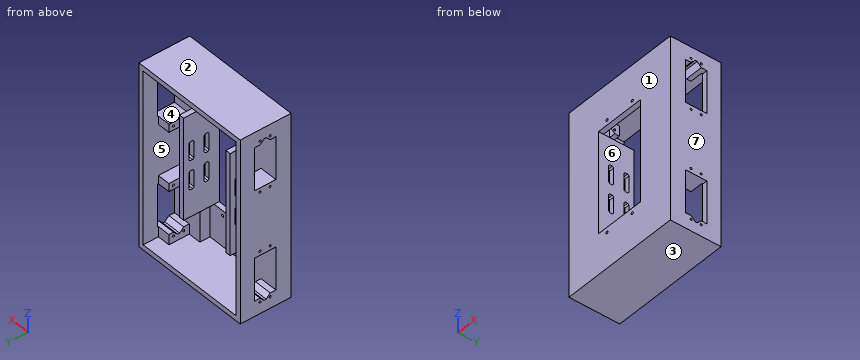
```python
from build123d import *

# Parameters (mm, degrees)
SKETCH1_W               = 120
SKETCH1_H               = 180
BOSS_EXTRUDE1_DEPTH     = 50
SHELL1_T                = -5
SKETCH2_W               = 5
SKETCH2_H               = 100
BOSS_EXTRUDE2_DEPTH     = 30
SKETCH3_W               = 25
SKETCH3_H               = 60
BOSS_EXTRUDE3_DEPTH     = 30
CUT_EXTRUDE1_REACH      = 224.036
SKETCH4_R               = 1
SKETCH5_W               = 12.5
SKETCH5_H               = 60
CUT_EXTRUDE2_DEPTH      = 20
CUT_EXTRUDE4_DEPTH      = 10
SKETCH6_R               = 1.25
SKETCH6_W               = 50
SKETCH6_H               = 100
CUT_EXTRUDE3_DEPTH      = 10
MIRROR2_COPY_1_SKETCH_W = 25
MIRROR2_COPY_1_SKETCH_H = 60
MIRROR2_COPY_1_DEPTH    = 30
MIRROR2_COPY_2_REACH    = 224.036
MIRROR2_COPY_2_SKETCH_R = 1
MIRROR2_COPY_3_SKETCH_W = 12.5
MIRROR2_COPY_3_SKETCH_H = 60
MIRROR2_COPY_3_DEPTH    = 20
MIRROR2_COPY_4_DEPTH    = 10


with BuildPart() as part:
    # Sketch1 → Boss-Extrude1 (new body)
    with BuildSketch(Plane(origin=(0, 0, 0), x_dir=(1, 0, 0), z_dir=(0, 1, 0))):
        with Locations((0, 90)):
            Rectangle(SKETCH1_W, SKETCH1_H)
    extrude(amount=BOSS_EXTRUDE1_DEPTH)

    # Shell1
    shell1_openings = [part.faces().sort_by_distance(p)[0] for p in [
        (0, 50, -90),
    ]]
    offset(amount=SHELL1_T, openings=shell1_openings, kind=Kind.INTERSECTION)

    # Sketch2 → Boss-Extrude2 (add)
    with BuildSketch(Plane(origin=(0, 5, 0), x_dir=(1, 0, 0), z_dir=(0, 1, 0))):
        with Locations((-27.5, 90)):
            Rectangle(SKETCH2_W, SKETCH2_H)
        with Locations((27.5, 90)):
            Rectangle(SKETCH2_W, SKETCH2_H)
    extrude(amount=BOSS_EXTRUDE2_DEPTH)

    # Sketch3 → Boss-Extrude3 (add)
    with BuildSketch(Plane(origin=(0, 5, 0), x_dir=(1, 0, 0), z_dir=(0, 1, 0))):
        with Locations((-42.5, 35)):
            Rectangle(SKETCH3_W, SKETCH3_H)
    boss_extrude3 = extrude(amount=BOSS_EXTRUDE3_DEPTH)

    # Cut-Extrude1: up to this face of the body (flat: up to its plane)
    cut_extrude1_end = Plane(part.part.faces().sort_by_distance((-30, 20, -102.5))[0])
    # Sketch4 → Cut-Extrude1 (cut, up to the picked face)
    with BuildSketch(Plane.ZY.offset(60), mode=Mode.PRIVATE) as cut_extrude1_sk1:
        with Locations((-61, 30.5)):
            Circle(SKETCH4_R)
    cut_extrude1_tool1 = split(extrude(cut_extrude1_sk1.sketch, amount=-CUT_EXTRUDE1_REACH, mode=Mode.PRIVATE), bisect_by=cut_extrude1_end, keep=Keep.BOTH, mode=Mode.PRIVATE)
    # Sketch4 → Cut-Extrude1 (cut, up to the picked face)
    with BuildSketch(Plane.ZY.offset(60), mode=Mode.PRIVATE) as cut_extrude1_sk2:
        with Locations((-61, 20.5)):
            Circle(SKETCH4_R)
    cut_extrude1_tool2 = split(extrude(cut_extrude1_sk2.sketch, amount=-CUT_EXTRUDE1_REACH, mode=Mode.PRIVATE), bisect_by=cut_extrude1_end, keep=Keep.BOTH, mode=Mode.PRIVATE)
    # Sketch4 → Cut-Extrude1 (cut, up to the picked face)
    with BuildSketch(Plane.ZY.offset(60), mode=Mode.PRIVATE) as cut_extrude1_sk3:
        with Locations((-11.220773398, 30.5)):
            Circle(SKETCH4_R)
    cut_extrude1_tool3 = split(extrude(cut_extrude1_sk3.sketch, amount=-CUT_EXTRUDE1_REACH, mode=Mode.PRIVATE), bisect_by=cut_extrude1_end, keep=Keep.BOTH, mode=Mode.PRIVATE)
    # Sketch4 → Cut-Extrude1 (cut, up to the picked face)
    with BuildSketch(Plane.ZY.offset(60), mode=Mode.PRIVATE) as cut_extrude1_sk4:
        with Locations((-11.220773398, 20.5)):
            Circle(SKETCH4_R)
    cut_extrude1_tool4 = split(extrude(cut_extrude1_sk4.sketch, amount=-CUT_EXTRUDE1_REACH, mode=Mode.PRIVATE), bisect_by=cut_extrude1_end, keep=Keep.BOTH, mode=Mode.PRIVATE)
    # Sketch4 → Cut-Extrude1 (cut, up to the picked face)
    with BuildSketch(Plane.ZY.offset(60), mode=Mode.PRIVATE) as cut_extrude1_sk5:
        Polygon((-57, 15), (-15, 15), (-15, 20.5), (-11, 24.5), (-11, 26.5), (-15, 30.5), (-15, 36), (-57, 36), align=None)
    cut_extrude1_tool5 = split(extrude(cut_extrude1_sk5.sketch, amount=-CUT_EXTRUDE1_REACH, mode=Mode.PRIVATE), bisect_by=cut_extrude1_end, keep=Keep.BOTH, mode=Mode.PRIVATE)
    cut_extrude1_1 = cut_extrude1_tool1.solids().sort_by(Axis((-60, 30.5, -61), (1, 0, 0)))[0]
    add(cut_extrude1_1, mode=Mode.SUBTRACT)
    cut_extrude1_2 = cut_extrude1_tool2.solids().sort_by(Axis((-60, 20.5, -61), (1, 0, 0)))[0]
    add(cut_extrude1_2, mode=Mode.SUBTRACT)
    cut_extrude1_3 = cut_extrude1_tool3.solids().sort_by(Axis((-60, 30.5, -11.220773), (1, 0, 0)))[0]
    add(cut_extrude1_3, mode=Mode.SUBTRACT)
    cut_extrude1_4 = cut_extrude1_tool4.solids().sort_by(Axis((-60, 20.5, -11.220773), (1, 0, 0)))[0]
    add(cut_extrude1_4, mode=Mode.SUBTRACT)
    cut_extrude1_5 = cut_extrude1_tool5.solids().sort_by(Axis((-60, 25.5, -35.402502), (1, 0, 0)))[0]
    add(cut_extrude1_5, mode=Mode.SUBTRACT)
    cut_extrude1 = cut_extrude1_1 + cut_extrude1_2 + cut_extrude1_3 + cut_extrude1_4 + cut_extrude1_5  # Cut-Extrude1 as one shape, for the pattern or mirror that repeats it

    # Sketch5 → Cut-Extrude2 (cut)
    with BuildSketch(Plane(origin=(0, 35, 0), x_dir=(1, 0, 0), z_dir=(0, 1, 0))):
        with Locations((-36.25, 35)):
            Rectangle(SKETCH5_W, SKETCH5_H)
    cut_extrude2 = extrude(amount=-CUT_EXTRUDE2_DEPTH, mode=Mode.SUBTRACT)

    # Sketch7 → Cut-Extrude4 (cut)
    with BuildSketch(Plane(origin=(-25, 0, 0), x_dir=(0, 0, -1), z_dir=(1, 0, 0))):
        Polygon((66.5, 28.75), (67.75, 30), (83.75, 30), (85, 28.75), (85, 26.25), (83.75, 25), (67.75, 25), (66.5, 26.25), align=None)
        Polygon((66.5, 13.75), (67.75, 15), (83.75, 15), (85, 13.75), (85, 11.25), (83.75, 10), (67.75, 10), (66.5, 11.25), align=None)
    cut_extrude4 = extrude(amount=-CUT_EXTRUDE4_DEPTH, mode=Mode.SUBTRACT)

    # Sketch6 → Cut-Extrude3 (cut)
    with BuildSketch(Plane(origin=(0, 5, 0), x_dir=(1, 0, 0), z_dir=(0, 1, 0))):
        with Locations(Location((-15, 145, 0), (0, 0, 270))):
            Circle(SKETCH6_R)
        with Locations(Location((15, 145, 0), (0, 0, 90))):
            Circle(SKETCH6_R)
        with Locations(Location((15, 35, 0), (0, 0, 270))):
            Circle(SKETCH6_R)
        with Locations(Location((-15, 35, 0), (0, 0, 90))):
            Circle(SKETCH6_R)
        with Locations((0, 90)):
            Rectangle(SKETCH6_W, SKETCH6_H)
    extrude(amount=-CUT_EXTRUDE3_DEPTH, mode=Mode.SUBTRACT)

    # Mirror1: Boss-Extrude3, Cut-Extrude1, Cut-Extrude2 across plane
    add(boss_extrude3.mirror(Plane(origin=(0, 0, 0), x_dir=(0, 0, 1), z_dir=(1, 0, 0))))
    add(cut_extrude1.mirror(Plane(origin=(0, 0, 0), x_dir=(0, 0, 1), z_dir=(1, 0, 0))), mode=Mode.SUBTRACT)
    add(cut_extrude2.mirror(Plane(origin=(0, 0, 0), x_dir=(0, 0, 1), z_dir=(1, 0, 0))), mode=Mode.SUBTRACT)

    # Mirror3: Cut-Extrude4 across plane
    add(cut_extrude4.mirror(Plane(origin=(0, 0, 0), x_dir=(0, 0, 1), z_dir=(1, 0, 0))), mode=Mode.SUBTRACT)

    # Mirror2: Boss-Extrude3, Cut-Extrude1, Cut-Extrude2, Cut-Extrude4 across plane
    add(boss_extrude3.mirror(Plane(origin=(0, 0, -90), x_dir=(1, 0, 0), z_dir=(0, 0, -1))))
    add(cut_extrude1.mirror(Plane(origin=(0, 0, -90), x_dir=(1, 0, 0), z_dir=(0, 0, -1))), mode=Mode.SUBTRACT)
    add(cut_extrude2.mirror(Plane(origin=(0, 0, -90), x_dir=(1, 0, 0), z_dir=(0, 0, -1))), mode=Mode.SUBTRACT)
    add(cut_extrude4.mirror(Plane(origin=(0, 0, -90), x_dir=(1, 0, 0), z_dir=(0, 0, -1))), mode=Mode.SUBTRACT)

    # Mirror2 copy 1 sketch → Mirror2 copy 1 (add)
    with BuildSketch(Plane(origin=(0, 5, -180), x_dir=(-1, 0, 0), z_dir=(0, 1, 0))):
        with Locations((-42.5, 35)):
            Rectangle(MIRROR2_COPY_1_SKETCH_W, MIRROR2_COPY_1_SKETCH_H)
    extrude(amount=MIRROR2_COPY_1_DEPTH)

    # Mirror2 copy 2: up to this face of the body (flat: up to its plane)
    mirror2_copy_2_end = Plane(part.part.faces().sort_by_distance((30, 20, -77.5))[0])
    # Mirror2 copy 2 sketch → Mirror2 copy 2 (cut, up to the picked face)
    with BuildSketch(Plane(origin=(60, 0, -180), x_dir=(0, 0, -1), z_dir=(1, 0, 0)), mode=Mode.PRIVATE) as mirror2_copy_2_sk1:
        with Locations((-61, 30.5)):
            Circle(MIRROR2_COPY_2_SKETCH_R)
    mirror2_copy_2_tool1 = split(extrude(mirror2_copy_2_sk1.sketch, amount=-MIRROR2_COPY_2_REACH, mode=Mode.PRIVATE), bisect_by=mirror2_copy_2_end, keep=Keep.BOTH, mode=Mode.PRIVATE)
    # Mirror2 copy 2 sketch → Mirror2 copy 2 (cut, up to the picked face)
    with BuildSketch(Plane(origin=(60, 0, -180), x_dir=(0, 0, -1), z_dir=(1, 0, 0)), mode=Mode.PRIVATE) as mirror2_copy_2_sk2:
        with Locations((-61, 20.5)):
            Circle(MIRROR2_COPY_2_SKETCH_R)
    mirror2_copy_2_tool2 = split(extrude(mirror2_copy_2_sk2.sketch, amount=-MIRROR2_COPY_2_REACH, mode=Mode.PRIVATE), bisect_by=mirror2_copy_2_end, keep=Keep.BOTH, mode=Mode.PRIVATE)
    # Mirror2 copy 2 sketch → Mirror2 copy 2 (cut, up to the picked face)
    with BuildSketch(Plane(origin=(60, 0, -180), x_dir=(0, 0, -1), z_dir=(1, 0, 0)), mode=Mode.PRIVATE) as mirror2_copy_2_sk3:
        with Locations((-11.220773398, 30.5)):
            Circle(MIRROR2_COPY_2_SKETCH_R)
    mirror2_copy_2_tool3 = split(extrude(mirror2_copy_2_sk3.sketch, amount=-MIRROR2_COPY_2_REACH, mode=Mode.PRIVATE), bisect_by=mirror2_copy_2_end, keep=Keep.BOTH, mode=Mode.PRIVATE)
    # Mirror2 copy 2 sketch → Mirror2 copy 2 (cut, up to the picked face)
    with BuildSketch(Plane(origin=(60, 0, -180), x_dir=(0, 0, -1), z_dir=(1, 0, 0)), mode=Mode.PRIVATE) as mirror2_copy_2_sk4:
        with Locations((-11.220773398, 20.5)):
            Circle(MIRROR2_COPY_2_SKETCH_R)
    mirror2_copy_2_tool4 = split(extrude(mirror2_copy_2_sk4.sketch, amount=-MIRROR2_COPY_2_REACH, mode=Mode.PRIVATE), bisect_by=mirror2_copy_2_end, keep=Keep.BOTH, mode=Mode.PRIVATE)
    # Mirror2 copy 2 sketch → Mirror2 copy 2 (cut, up to the picked face)
    with BuildSketch(Plane(origin=(60, 0, -180), x_dir=(0, 0, -1), z_dir=(1, 0, 0)), mode=Mode.PRIVATE) as mirror2_copy_2_sk5:
        Polygon((-57, 15), (-15, 15), (-15, 20.5), (-11, 24.5), (-11, 26.5), (-15, 30.5), (-15, 36), (-57, 36), align=None)
    mirror2_copy_2_tool5 = split(extrude(mirror2_copy_2_sk5.sketch, amount=-MIRROR2_COPY_2_REACH, mode=Mode.PRIVATE), bisect_by=mirror2_copy_2_end, keep=Keep.BOTH, mode=Mode.PRIVATE)
    add(mirror2_copy_2_tool1.solids().sort_by(Axis((60, 30.5, -119), (-1, 0, 0)))[0], mode=Mode.SUBTRACT)
    add(mirror2_copy_2_tool2.solids().sort_by(Axis((60, 20.5, -119), (-1, 0, 0)))[0], mode=Mode.SUBTRACT)
    add(mirror2_copy_2_tool3.solids().sort_by(Axis((60, 30.5, -168.779227), (-1, 0, 0)))[0], mode=Mode.SUBTRACT)
    add(mirror2_copy_2_tool4.solids().sort_by(Axis((60, 20.5, -168.779227), (-1, 0, 0)))[0], mode=Mode.SUBTRACT)
    add(mirror2_copy_2_tool5.solids().sort_by(Axis((60, 25.5, -144.597498), (-1, 0, 0)))[0], mode=Mode.SUBTRACT)

    # Mirror2 copy 3 sketch → Mirror2 copy 3 (cut)
    with BuildSketch(Plane(origin=(0, 35, -180), x_dir=(-1, 0, 0), z_dir=(0, 1, 0))):
        with Locations((-36.25, 35)):
            Rectangle(MIRROR2_COPY_3_SKETCH_W, MIRROR2_COPY_3_SKETCH_H)
    extrude(amount=-MIRROR2_COPY_3_DEPTH, mode=Mode.SUBTRACT)

    # Mirror2 copy 4 sketch → Mirror2 copy 4 (cut)
    with BuildSketch(Plane(origin=(25, 0, -180), x_dir=(0, 0, 1), z_dir=(-1, 0, 0))):
        Polygon((66.5, 28.75), (67.75, 30), (83.75, 30), (85, 28.75), (85, 26.25), (83.75, 25), (67.75, 25), (66.5, 26.25), align=None)
        Polygon((66.5, 13.75), (67.75, 15), (83.75, 15), (85, 13.75), (85, 11.25), (83.75, 10), (67.75, 10), (66.5, 11.25), align=None)
    extrude(amount=-MIRROR2_COPY_4_DEPTH, mode=Mode.SUBTRACT)


solid = part.part
```
CAD build for the part. Positions are in the model's coordinates, mm. Face numbers are marked on the shaded views. A direction names the side the tool comes from. Round coordinates to 2 decimals unless told otherwise and drop trailing zeros. Loops run counter-clockwise (first coordinate to the right, second up) from the corner with the lowest first, then second, coordinate; pieces in that order, holes last. Notation, with made-up numbers: (-33.75, 77) - (25.25, 77) arc R10 ccw to (25.25, 83) - close; hole circle Ø10 at (-17.75, 67.25). An arc over 180 degrees is marked (long way). Return JSON: item names as keys, results as strings. Group by question number.
Q1. Band-saw the part on A-A on z = -73. Give the number of separate pieces and of enclosed holes in the cut face, plus the area to 3 significant figures.
Q2. Band-saw the part on B-B on x = -5.5. Give the cut face in (y, z).
Q3. Band-saw the part on C-C on z = -24.5. Give the cut face in (x, y).
Q4. Two-plate mould, pull along Z, no slides. Class the marked faces 1, 2, 3 and 4: +Z half, -Z half, draft (parallel to the pull), parting line (faces both ways), or undercut.
Q5. Drill centre lines: line 1 along X through (y, z) = (2, -35); line 2 along Z through (x, y) = (28.5, 27); line 3 along Y through (x, z) = (26, -98). Where is each one in solid material? Low to high. Write a range as [from, to].
Q6. Flat gauge pins, fed straight in: pin 1 Ø12 at (x, z) = (39.5, -48) entering from -Y; pin 2 Ø12 at (x, z) = (-27, -119.5) entering from +Y; pin 3 Ø1.8 at (y, z) = (20.5, -11.22) entering from -X. Where does each tip first touch, or does it go through?
Q7. Band-saw the part on D-D on y = 7.5. Give the cut face in (x, z), plus the area to 3 significant figures.
Q8. Tool access for the marked faces 5, 6 and 7: list every direction of +Z, -Z, +X, -X, +Y, -Y with a clear straight run to the whole face (end or side of a thin tool).
Solutions:
{
 "1": {"separate pieces": "6", "enclosed holes": "0", "area": "1,000 mm^2"},
 "2": {"outline": "(0, -180) - (50, -180) - (50, -175) - (5, -175) - (5, -140) - (0, -140) - close; (0, -40) - (5, -40) - (5, -5) - (50, -5) - (50, 0) - (0, 0) - close"},
 "3": {"outline": "(-60, 0) - (60, 0) - (60, 15) - (30, 15) - (30, 5) - (-30, 5) - (-30, 15) - (-60, 15) - close; (-60, 36) - (-55, 36) - (-55, 50) - (-60, 50) - close; (55, 36) - (60, 36) - (60, 50) - (55, 50) - close"},
 "4": {"face 1": "draft", "face 2": "+Z half", "face 3": "-Z half", "face 4": "undercut"},
 "5": {"line 1": "x = [-60, -16.25], [-13.75, 13.75], [16.25, 60]", "line 2": "z = [-180, -175], [-140, -113.5], [-95, -85], [-66.5, -40], [-5, 0]", "line 3": "y = [0, 10], [15, 25], [30, 35]"},
 "6": {"pin 1": "stops at y = 0", "pin 2": "stops at y = 35", "pin 3": "passes through"},
 "7": {"outline": "(-60, -180) - (60, -180) - (60, 0) - (-60, 0) - close; hole (-55, -115) - (-30, -115) - (-30, -65) - (-55, -65) - close; hole (-30, -175) - (30, -175) - (30, -140) - (25, -140) - (25, -40) - (30, -40) - (30, -5) - (-30, -5) - (-30, -40) - (-25, -40) - (-25, -140) - (-30, -140) - close; hole (30, -115) - (55, -115) - (55, -65) - (30, -65) - close", "area": "9,900 mm^2"},
 "8": {"face 5": "+Y", "face 6": "+Y, -Y", "face 7": "+Z, -Z, +X, +Y, -Y"}
}
